```python
from build123d import *

# Parameters (mm, degrees)
ESQUISSE1_W             = 76
ESQUISSE1_H             = 76
BOSS_EXTRU_1_DEPTH      = 6
ESQUISSE3_W             = 76
ESQUISSE3_H             = 50
BOSS_EXTRU_2_DEPTH      = 6
ESQUISSE4_W             = 50
ESQUISSE4_H             = 82
BOSS_EXTRU_3_DEPTH      = 6
ESQUISSE5_W             = 50
ESQUISSE5_H             = 82
BOSS_EXTRU_4_DEPTH      = 6
ESQUISSE6_W             = 88
ESQUISSE6_H             = 50
BOSS_EXTRU_5_DEPTH      = 6
ESQUISSE8_W             = 54
ESQUISSE8_H             = 7
BOSS_EXTRU_6_DEPTH      = 26
ESQUISSE9_W             = 54
ESQUISSE9_H             = 6
BOSS_EXTRU_7_DEPTH      = 40.5
ESQUISSE11_W            = 54
ESQUISSE11_H            = 7
BOSS_EXTRU_8_DEPTH      = 26
BOSS_EXTRU_10_DEPTH     = 54
ESQUISSE13_R            = 1
ENL_V_MAT_EXTRU_1_DEPTH = 100


with BuildPart() as part:
    # Esquisse1 → Boss.-Extru.1 (new body)
    with BuildSketch(Plane.XY):
        with Locations((-3, -3)):
            Rectangle(ESQUISSE1_W, ESQUISSE1_H)
    extrude(amount=BOSS_EXTRU_1_DEPTH)

    # Esquisse3 → Boss.-Extru.2 (add)
    with BuildSketch(Plane(origin=(0, -41, 0), x_dir=(-1, 0, 0), z_dir=(0, -1, 0))):
        with Locations((3, -25)):
            Rectangle(ESQUISSE3_W, ESQUISSE3_H)
    extrude(amount=BOSS_EXTRU_2_DEPTH)

    # Esquisse4 → Boss.-Extru.3 (add)
    with BuildSketch(Plane.ZY.offset(41)):
        with Locations((25, -6)):
            Rectangle(ESQUISSE4_W, ESQUISSE4_H)
    extrude(amount=BOSS_EXTRU_3_DEPTH)

    # Esquisse5 → Boss.-Extru.4 (add)
    with BuildSketch(Plane(origin=(35, 0, 0), x_dir=(0, 0, -1), z_dir=(1, 0, 0))):
        with Locations((-25, -6)):
            Rectangle(ESQUISSE5_W, ESQUISSE5_H)
    extrude(amount=BOSS_EXTRU_4_DEPTH)

    # Esquisse6 → Boss.-Extru.5 (add)
    with BuildSketch(Plane(origin=(0, 35, 0), x_dir=(1, 0, 0), z_dir=(0, 1, 0))):
        with Locations((-3, -25)):
            Rectangle(ESQUISSE6_W, ESQUISSE6_H)
    extrude(amount=BOSS_EXTRU_5_DEPTH)

    # Esquisse8 → Boss.-Extru.6 (add)
    with BuildSketch(Plane(origin=(0, 0, 0), x_dir=(-1, 0, 0), z_dir=(0, 0, -1))):
        with Locations((3, 32.065521745)):
            Rectangle(ESQUISSE8_W, ESQUISSE8_H)
    extrude(amount=BOSS_EXTRU_6_DEPTH)

    # Esquisse9 → Boss.-Extru.7 (add)
    with BuildSketch(Plane(origin=(0, 28.565521745, 0), x_dir=(-1, 0, 0), z_dir=(0, -1, 0))):
        with Locations((3, 23)):
            Rectangle(ESQUISSE9_W, ESQUISSE9_H)
    extrude(amount=BOSS_EXTRU_7_DEPTH)

    # Esquisse11 → Boss.-Extru.8 (add)
    with BuildSketch(Plane(origin=(0, 0, -26), x_dir=(-1, 0, 0), z_dir=(0, 0, -1))):
        with Locations((3, -15.434478255)):
            Rectangle(ESQUISSE11_W, ESQUISSE11_H)
    extrude(amount=-BOSS_EXTRU_8_DEPTH)

    # Esquisse12 → Boss.-Extru.10 (add)
    with BuildSketch(Plane(origin=(24, 0, 0), x_dir=(0, 0, -1), z_dir=(1, 0, 0))):
        Polygon((26, -18.934478255), (0, -18.934478255), (0, -30.364478255), align=None)
        Polygon((0, 35.565521745), (26, 35.565521745), (0, 41), align=None)
    extrude(amount=-BOSS_EXTRU_10_DEPTH)

    # Esquisse13 → Enlèv. mat.-Extru.1 (cut)
    with BuildSketch(Plane(origin=(0, -47, 0), x_dir=(-1, 0, 0), z_dir=(0, -1, 0))):
        with Locations(Location((-26, -40, 0), (0, 0, 90))):
            Circle(ESQUISSE13_R)
        with Locations(Location((32, -40, 0), (0, 0, 90))):
            Circle(ESQUISSE13_R)
    extrude(amount=-ENL_V_MAT_EXTRU_1_DEPTH, mode=Mode.SUBTRACT)


solid = part.part
```
Can you work these out from the model? Positions are in its coordinate system, mm. A direction names the side the tool comes from. Round coordinates to 2 decimals unless told otherwise and drop trailing zeros. Loops run counter-clockwise (first coordinate to the right, second up) from the corner with the lowest first, then second, coordinate; pieces in that order, holes last. Notation, with made-up numbers: (-12, -9) -> (41, -9) arc R22 cw to (41, 5) -> close; hole circle Ø9 at (75, 3.25). An arc over 180 degrees is marked (long way). One line per item, written item: value. Start each with the question number.
1. For faces 1 (the flat face through (-47, -4, 25)), 2 (the flat face through (-2, -41, 28)), 3 (the flat face through (-3, -11.934, -10)), 4 (the flat face through (24, 6, -21)), which set-ups out of +Z, -Z, +X, -X, +Y, -Y let a thin tool reach every point of the face, with its end or its side?
2. If we section it at C-C, the plane y = 7.5: Write out the boundary of the cut face in (x, z).
3. For pin 1 (21 mm diameter, centred on y = 22.5, z = -11, fed in from +X); pin 2 (1.8 mm diameter, centred on x = 26, z = 40, fed in from +Y); pin 3 (2.5 mm diameter, centred on x = -32, z = 40, fed in from -Y); pin 4 (10 mm diameter, centred on x = 8.5, z = -11.5, fed in from -Y), each with a flat end and sliding along its axis, tell me the tip position at first contact or that it passes through.
4. If we mould it in two halves opening along Z, with no side actions, what happens to faces 5 (the flat face through (-4, -4, 0)), 6 (the flat face through (-30, 6, -21)), 7 (the flat face through (-2.622, 38.245, -13.182)), 8 (the flat face through (-3, 9, -20))? For each: pulls with the +Z half, pulls with the -Z half, needs draft (parallel to the pull), parting line crosses it, or undercut.
5. If we section it at A-A, the plane x = -5.5: Write out the boundary of the cut face in (y, z), then the cut area to 3 significant figures.
6. If we section it at B-B, the plane z = -3: Write out the boundary of the cut face in (x, y).
7. If I drill on probe 1 along X at (y, z) = (-42.45, 40); probe 2 along Y at (x, z) = (20, 41); probe 3 along Z at (x, y) = (15, 4), over which ranges is the centre line in solid material (lowest first)?
8. If we section it at D-D, the plane z = 43: Write out the boundary of the cut face in (x, y).
Calculated:
1. face 1: +Z, -Z, -X, +Y, -Y
1. face 2: +Z
1. face 3: +X, -X
1. face 4: -Z, +X, +Y, -Y
2. outline: (-47, 0) -> (41, 0) -> (41, 50) -> (35, 50) -> (35, 6) -> (-41, 6) -> (-41, 50) -> (-47, 50) -> close; (-30, -26) -> (24, -26) -> (24, -20) -> (-30, -20) -> close
3. pin 1: stops at x = 24
3. pin 2: passes through
3. pin 3: stops at y = -47
3. pin 4: stops at y = -27.51
4. face 5: undercut
4. face 6: needs draft
4. face 7: pulls with the -Z half
4. face 8: undercut
5. outline: (-47, 0) -> (-30.36, 0) -> (-18.93, -26) -> (35.57, -26) -> (41, 0) -> (41, 50) -> (35, 50) -> (35, 6) -> (-41, 6) -> (-41, 50) -> (-47, 50) -> close; hole (-11.93, -20) -> (28.57, -20) -> (28.57, 0) -> (-11.93, 0) -> close
5. area: 1,880 mm²
6. outline: (-30, -29.05) -> (24, -29.05) -> (24, -11.93) -> (-30, -11.93) -> close; (-30, 28.57) -> (24, 28.57) -> (24, 40.37) -> (-30, 40.37) -> close
7. probe 1: x = -47 to -33, -31 to 25, 27 to 41
7. probe 2: y = -47 to -41, 35 to 41
7. probe 3: z = -26 to -20, 0 to 6
8. outline: (-47, -47) -> (41, -47) -> (41, 41) -> (-47, 41) -> close; hole (-41, -41) -> (35, -41) -> (35, 35) -> (-41, 35) -> close
